Model file for the job. Use its own axes, mm. A direction names the side the tool comes from. Coordinates: 2 decimals unless noted, no trailing zeros. Order: outer loops, then holes, each group sorted by start corner. A loop starts at its lowest first (then second) coordinate and runs counter-clockwise, first axis right, second up. Notation, with made-up numbers: (54.25, -6.75) -> (95.25, -6.75) arc R32 cw to (95.25, 27.25) -> close; hole circle Ø5 at (85.5, 48.25). An arc over 180 degrees is marked (long way). Write item = value, one per line. Start each with the question number.
Q1. 3-axis set-ups, long thin cutter, end or side, ignore diameter. For faces 4 (the face through (-25, -5, 0)), 5 (the face through (-25, -25, 30)), 6 (the face through (-15.1, -22.1, 6.8)), 7 (the face through (-8, -10, 7)), 8 (the face through (-14.9, -24.9, 23.2)): which of +Z, -Z, +X, -X, +Y, -Y reach the whole face in a straight line?
Q2. Mould opens along Y. For faces 1 (the face through (-22.36, -14.93, 23.43)), 2 (the face through (-5, -5, 30)), 3 (the face through (-15, -30, 15)) say: +Y half, -Y half, draft (parallel to the pull), parting line (faces both ways), or undercut.
Q3. Cut at D-D, the plane z = 10. List the corners of the cut face in (x, y), plus the area to 3 significant figures.
Q4. Wall check: line 1 (X direction, y = -13.25, z = 17.5) (3 decimals); line 2 (Y direction, x = -25.25, z = 9.5) (3 decimals); line 3 (X direction, y = -2.75, z = 19). Give the ranges that are in metal, low to high. Write a range as from..to.
Q5. Cut at A-A, the plane z = 2. List the corners of the cut face in (x, y), plus the area to 3 significant figures.
Q6. Cut at B-B, the plane x = -22.5. List the corners of the cut face in (y, z).
Q7. Cut at C-C, the plane y = -6.5. List the corners of the cut face in (x, z), plus the area to 3 significant figures.
from build123d import *

# Parameters (mm, degrees)
F1_DEPTH = 30
F3_DEPTH = 30.001


with BuildPart() as f1:
    # F0 (on Front) → F1 (new body)
    with BuildSketch(Plane.XZ):
        Polygon((-30, 30), (-30, 0), (-20, 0), (-20, 13.333333), (-10, 0), (0, 0), (0, 30), (-10, 30), (-10, 16.666667), (-20, 30), align=None)
    extrude(amount=F1_DEPTH)

    # F2 (on face) → F3 (cut, through all)
    with BuildSketch(Plane(origin=(-30, 0, 0), x_dir=(0, -1, 0), z_dir=(-1, 0, 0))):
        Polygon((20, 30), (10, 30), (20, 16.666667), align=None)
        Polygon((10, 13.333333), (10, 0), (20, 0), align=None)
    extrude(amount=-F3_DEPTH, mode=Mode.SUBTRACT)


solid = f1.part
Here are the results:
q1.face_4 = -Z, +X, -X, +Y, -Y
q1.face_5 = +Z, +X, -X, +Y, -Y
q1.face_6 = -Z, +Y, -Y
q1.face_7 = -Z, +X, -X
q1.face_8 = +Z, +Y, -Y
q2.face_1 = undercut
q2.face_2 = draft
q2.face_3 = -Y half
q3.outline = (-30, -30) -> (-20, -30) -> (-20, -12.5) -> (-30, -12.5) -> close; (-30, -10) -> (-20, -10) -> (-20, 0) -> (-30, 0) -> close; (-17.5, -30) -> (0, -30) -> (0, -12.5) -> (-17.5, -12.5) -> close; (-17.5, -10) -> (0, -10) -> (0, 0) -> (-17.5, 0) -> close
q3.area = 756 mm²
q4.line_1 = -30..-10.625, -10..0
q4.line_2 = -30..-12.875, -10..0
q4.line_3 = -30..-11.75, -10..0
q5.outline = (-30, -30) -> (-20, -30) -> (-20, -18.5) -> (-30, -18.5) -> close; (-30, -10) -> (-20, -10) -> (-20, 0) -> (-30, 0) -> close; (-11.5, -30) -> (0, -30) -> (0, -18.5) -> (-11.5, -18.5) -> close; (-11.5, -10) -> (0, -10) -> (0, 0) -> (-11.5, 0) -> close
q5.area = 462 mm²
q6.outline = (-30, 0) -> (-20, 0) -> (-10, 13.33) -> (-10, 0) -> (0, 0) -> (0, 30) -> (-10, 30) -> (-20, 16.67) -> (-20, 30) -> (-30, 30) -> close
q7.outline = (-30, 0) -> (-20, 0) -> (-20, 13.33) -> (-10, 0) -> (0, 0) -> (0, 30) -> (-10, 30) -> (-10, 16.67) -> (-20, 30) -> (-30, 30) -> close
q7.area = 767 mm²
